CAD build for the part. Positions are in the model's coordinates, mm. Face numbers are marked on the shaded views. Give positions to 0.01 mm unless a question says otherwise; leave off trailing zeros. Write each loop counter-clockwise with the first axis right and the second up, starting at its lowest first coordinate (ties: lowest second). Pieces come first, ordered by that corner, then holes. Notation, with made-up numbers: (75, -36.75) - (118, -36.75) arc R5 cw to (118, -29.75) - close; hole circle Ø4 at (47, 20). An arc over 180 degrees is marked (long way). Put each result on its own line as item: value. Start each with the question number.
1. Cut at A-A on y = 1.75. List the corners of the cut face in (x, z) (1 decimal), and give its area (3 significant figures).
2. Mould opens along X. For the marked faces 1, 2, 3 and 4 say: +X half, -X half, draft (parallel to the pull), parting line (faces both ways), or undercut.
3. Cut at C-C on z = 0. List the corners of the cut face in (x, y), and give its area (3 significant figures).
4. Wall check: line 1 (X direction, y = 1.85, z = 0); line 2 (Z direction, x = 0, y = 3.35). Give the ranges that are in metal, low to high.
5. Drop flat-ended pins along their axis: pin 1 (2 mm diameter, centred on x = -3.5, y = 1.5, fed in from -Z); pin 2 (1.4 mm diameter, centred on x = 0, z = 0, fed in from -Y); pin 3 (1.5 mm diameter, centred on y = 1, z = 2.5, fed in from +X). Give the stop position or say it passes through.
6. Cut at B-B on x = 0. List the corners of the cut face in (y, z), and give its area (3 significant figures).
from build123d import *


with BuildPart() as part:
    # Sketch1 → Revolve1 (revolve)
    with BuildSketch(Plane.XY):
        with BuildLine():
            Line((-1.5494, 0), (-1.5494, 3.048))
            Line((-1.5494, 3.048), (-0.762, 3.048))
            Line((-0.762, 3.048), (-0.762, 4.064))
            Line((-0.762, 4.064), (0, 4.064))
            Line((0, 4.064), (0, 5.08))
            ThreePointArc((0, 5.08), (-2.074697908, 5.383049508), (-3.976029965, 6.266874616))
            ThreePointArc((-3.976029965, 6.266874616), (-4.495955195, 6.288948978), (-4.7625, 5.842))
            Line((-4.7625, 5.842), (-4.7625, 0))
            Line((-4.7625, 0), (-3.4925, 0))
            Line((-3.4925, 0), (-3.4925, 4.064))
            Line((-3.4925, 4.064), (-2.0574, 4.064))
            Line((-2.0574, 4.064), (-2.0574, 0))
            Line((-2.0574, 0), (-1.5494, 0))
        make_face()
    revolve(axis=Axis((0, 0, 0), (0, -1, 0)))


solid = part.part
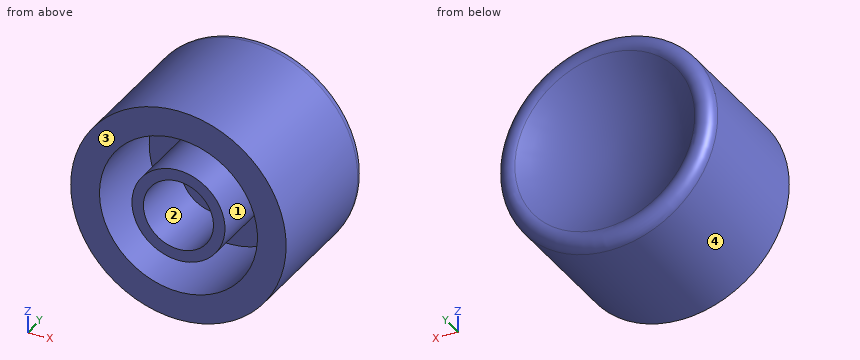
Report:
1. outline: circle Ø9.5 at (0, 0); circle Ø4.1 at (0, 0); hole circle Ø7 at (0, 0); hole circle Ø3.1 at (0, 0)
1. area: 38.7 mm²
2. face 1: undercut
2. face 2: undercut
2. face 3: draft
2. face 4: parting line
3. outline: (-4.76, 0) - (-3.49, 0) - (-3.49, 4.06) - (-2.06, 4.06) - (-2.06, 0) - (-1.55, 0) - (-1.55, 3.05) - (-0.76, 3.05) - (-0.76, 4.06) - (0.76, 4.06) - (0.76, 3.05) - (1.55, 3.05) - (1.55, 0) - (2.06, 0) - (2.06, 4.06) - (3.49, 4.06) - (3.49, 0) - (4.76, 0) - (4.76, 5.84) arc R0.51 ccw to (3.98, 6.27) arc R7.25 cw to (-3.98, 6.27) arc R0.51 ccw to (-4.76, 5.84) - close
3. area: 30.6 mm²
4. line 1: x = -4.76 to -3.49, -2.06 to -1.55, 1.55 to 2.06, 3.49 to 4.76
4. line 2: z = -4.76 to -3.49, -2.06 to -0.76, 0.76 to 2.06, 3.49 to 4.76
5. pin 1: stops at z = -4.05
5. pin 2: stops at y = 4.06
5. pin 3: stops at x = 4.43
6. outline: (0, -4.76) - (5.84, -4.76) arc R0.51 ccw to (6.27, -3.98) arc R7.25 cw to (6.27, 3.98) arc R0.51 ccw to (5.84, 4.76) - (0, 4.76) - (0, 3.49) - (4.06, 3.49) - (4.06, 2.06) - (0, 2.06) - (0, 1.55) - (3.05, 1.55) - (3.05, 0.76) - (4.06, 0.76) - (4.06, -0.76) - (3.05, -0.76) - (3.05, -1.55) - (0, -1.55) - (0, -2.06) - (4.06, -2.06) - (4.06, -3.49) - (0, -3.49) - close
6. area: 30.6 mm²
